Could you check a few things on this drawing? It's one solid part, dimensions in mm from its lowest x, y, z. A direction names the side the tool comes from. Round coordinates to 2 decimals unless told otherwise and drop trailing zeros. Write each loop counter-clockwise with the first axis right and the second up, starting at its lowest first coordinate (ties: lowest second). Pieces come first, ordered by that corner, then holes. Notation, with made-up numbers: (29, -1.75) -> (86, -1.75) arc R30 ccw to (86, 37.25) -> close; hole circle Ø3 at (15, 54). An arc over 180 degrees is marked (long way). Answer in a Markdown table with one row per item. Add a question column.
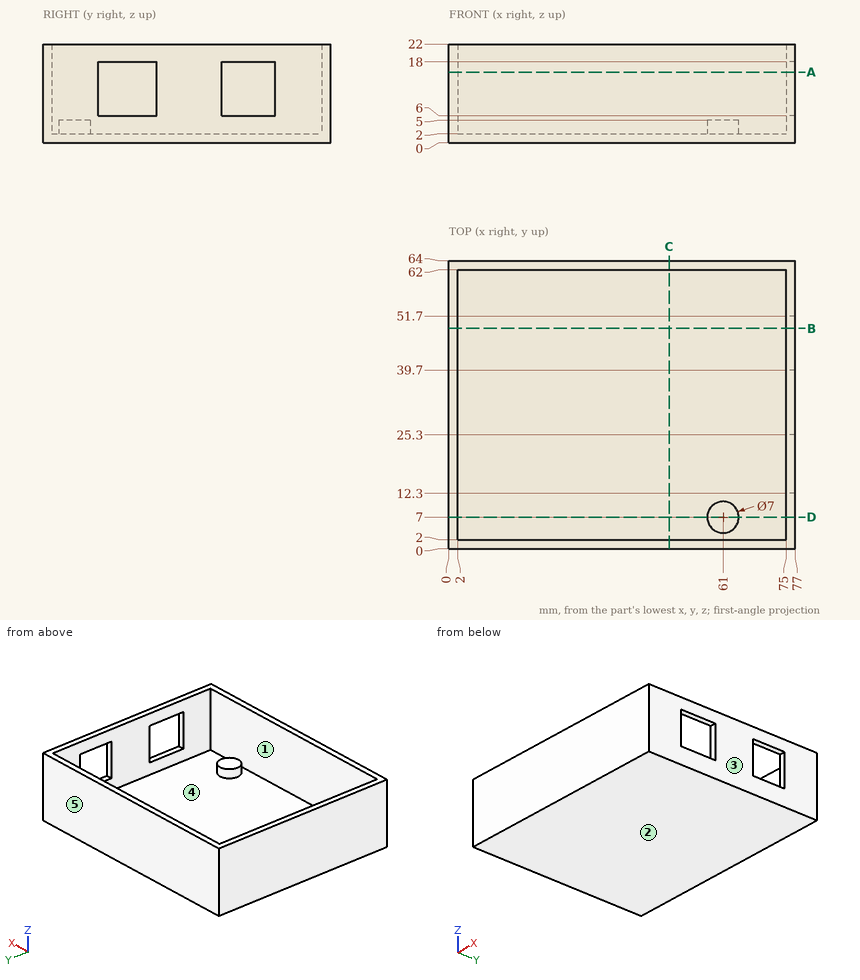
(1) On a 3-axis mill with a long thin cutter (end or side, diameter ignored), from which of +Z, -Z, +X, -X, +Y, -Y can I reach the whole of each face in a straight line? I mean the marked faces 1 and 2. Say none if no direction works.
(2) I need wall thicknesses on L1, parallel to X at y = 37.5, z = 17; L2, parallel to Y at x = 9, z = 8.5; L3, parallel to Z at x = 29.5, y = 23. Which ranges of each line are inside material? Lowest first, please.
(3) Suppose I cut it at B-B, the plane y = 49. Please give me the cut outline in (x, z).
(4) If we mould it in two halves opening along Y, with no side actions, what happens to the marked faces 3, 4 and 5? For each: pulls with the +Y half, pulls with the -Y half, needs draft (parallel to the pull), parting line crosses it, or undercut.
(5) Suppose I cut it at A-A, the plane z = 15.75. Please give me the cut outline in (x, y).
(6) For P1, Ø6, axis at x = 32, y = 56, coming from the +Z side; P2, Ø5.5, axis at x = 59.5, y = 8.5, coming from the +Z side, each with a flat end and sliding along its axis, tell me the tip position at first contact or that it passes through.
(7) Suppose I cut it at D-D, the plane y = 7. Please give me the cut outline in (x, z).
(8) Suppose I cut it at C-C, the plane x = 49. Please give me the cut outline in (y, z), then the cut area to 3 significant figures.
Response:
| question | item | result |
|---|---|---|
| 1 | face 1 | +Z |
| 1 | face 2 | -Z, +X, -X, +Y, -Y |
| 2 | L1 | 0 to 2, 75 to 77 |
| 2 | L2 | 0 to 2, 62 to 64 |
| 2 | L3 | 0 to 2 |
| 3 | outline | (0, 0) -> (77, 0) -> (77, 6) -> (75, 6) -> (75, 2) -> (2, 2) -> (2, 22) -> (0, 22) -> close; (75, 18) -> (77, 18) -> (77, 22) -> (75, 22) -> close |
| 4 | face 3 | needs draft |
| 4 | face 4 | undercut |
| 4 | face 5 | pulls with the +Y half |
| 5 | outline | (0, 0) -> (77, 0) -> (77, 12.3) -> (75, 12.3) -> (75, 2) -> (2, 2) -> (2, 62) -> (75, 62) -> (75, 51.7) -> (77, 51.7) -> (77, 64) -> (0, 64) -> close; (75, 25.3) -> (77, 25.3) -> (77, 39.7) -> (75, 39.7) -> close |
| 6 | P1 | z = 2 |
| 6 | P2 | z = 5 |
| 7 | outline | (0, 0) -> (77, 0) -> (77, 22) -> (75, 22) -> (75, 2) -> (64.5, 2) -> (64.5, 5) -> (57.5, 5) -> (57.5, 2) -> (2, 2) -> (2, 22) -> (0, 22) -> close |
| 8 | outline | (0, 0) -> (64, 0) -> (64, 22) -> (62, 22) -> (62, 2) -> (2, 2) -> (2, 22) -> (0, 22) -> close |
| 8 | area | 208 mm² |
